Read the model definition and answer for the solid it produces. Units are mm, in the model's axes. Face numbers are marked on the shaded views. A direction names the side the tool comes from. Coordinates: 2 decimals unless noted, no trailing zeros. Write each loop counter-clockwise with the first axis right and the second up, starting at its lowest first coordinate (ties: lowest second). Pieces come first, ordered by that corner, then holes.
(1) Section B-B on y = -23.5 is taken. Write down the section's boundary in (x, z).
(2) Given pin 1 (1.5 mm diameter, centred on x = -63, y = -18, fed in from -Z); pin 2 (9.5 mm diameter, centred on y = -42, z = 39, fed in from -X); pin 3 (5.5 mm diameter, centred on x = -64, y = -33, fed in from +Z); pin 4 (14.5 mm diameter, centred on x = -72, z = 50.5, fed in from -Y), each flat-ended and moving along its own axis, determine where each tip first touches the part or whether it passes through.
(3) Which of the six approach directions +Z, -Z, +X, -X, +Y, -Y give full straight-line access (tool end or side, diameter ignored) to the marked faces 1, 2, 3 and 4?
(4) Section A-A on y = -32 is taken. Write down the section's boundary in (x, z).
(5) Find the intervals of material crossed by probe 1 along X at (y, z) = (-6.5, 39); probe 2 along Y at (x, z) = (-41, 38); probe 3 along X at (y, z) = (-31.5, 32.5), in increasing order.
(6) Section C-C on y = -14 is taken. Write down the section's boundary in (x, z).
from build123d import *

# Parameters (mm, degrees)
F0_R     = 29.935911
F1_DEPTH = 25.4
F2_R     = 5.518892
F3_W     = 18.751926
F3_H     = 19.416006
F4_DEPTH = 25.4


with BuildPart() as f1:
    # F0 (on Front) → F1 (new body)
    with BuildSketch(Plane.XZ):
        with Locations((-61.485115, 39.142173)):
            Circle(F0_R)
    extrude(amount=F1_DEPTH)

    # F2
    f2_edges = [f1.edges().sort_by_distance(p)[0] for p in [
        (-91.421026, -25.4, 39.142173),
    ]]
    fillet(f2_edges, radius=F2_R)

    # F3 (on face) → F4 (join)
    with BuildSketch(Plane.XZ.offset(25.4)):
        with Locations((-62.324103, 37.501703)):
            Rectangle(F3_W, F3_H)
    extrude(amount=F4_DEPTH)


solid = f1.part
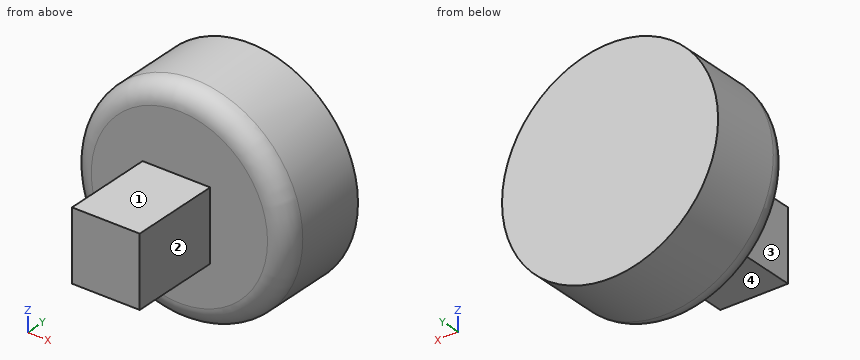
Response:
1. outline: circle Ø57.17 at (-61.49, 39.14)
2. pin 1: stops at z = 9.22
2. pin 2: stops at x = -71.7
2. pin 3: stops at z = 47.21
2. pin 4: stops at y = -50.8
3. face 1: +Z, +X, -X, -Y
3. face 2: +Z, -Z, +X, -Y
3. face 3: +Z, -Z, -X, -Y
3. face 4: -Z, +X, -X, -Y
4. outline: (-71.7, 27.79) - (-52.95, 27.79) - (-52.95, 47.21) - (-71.7, 47.21) - close
5. probe 1: x = -91.42 to -31.55
5. probe 2: y = -25.4 to 0
5. probe 3: x = -71.7 to -52.95
6. outline: circle Ø59.87 at (-61.49, 39.14)
